from build123d import *

# Parameters (mm, degrees)
ESQUISSE2_W        = 86
ESQUISSE2_H        = 25
ESQUISSE2_R        = 4.05
ESQUISSE2_R_2      = 1
ESQUISSE2_R_3      = 1.5
ESQUISSE2_W_2      = 5
ESQUISSE2_H_2      = 5
BOSS_EXTRU_1_DEPTH = 2
CONG_1_R           = 5


with BuildPart() as part:
    # Esquisse2 → Boss.-Extru.1 (new body)
    with BuildSketch(Plane(origin=(0, 0, 0), x_dir=(-1, 0, 0), z_dir=(0, 0, -1))):
        with Locations((-43, 0)):
            Rectangle(ESQUISSE2_W, ESQUISSE2_H)
        with Locations((-11, 0)):
            Circle(ESQUISSE2_R, mode=Mode.SUBTRACT)
        with Locations((-4, 0)):
            Circle(ESQUISSE2_R_2, mode=Mode.SUBTRACT)
        with Locations((-4.937822174, -3.5)):
            Circle(ESQUISSE2_R_2, mode=Mode.SUBTRACT)
        with Locations((-7.5, -6.062177826)):
            Circle(ESQUISSE2_R_2, mode=Mode.SUBTRACT)
        with Locations((-11, -7)):
            Circle(ESQUISSE2_R_2, mode=Mode.SUBTRACT)
        with Locations((-14.5, -6.062177826)):
            Circle(ESQUISSE2_R_2, mode=Mode.SUBTRACT)
        with Locations((-17.062177826, -3.5)):
            Circle(ESQUISSE2_R_2, mode=Mode.SUBTRACT)
        with Locations((-18, 0)):
            Circle(ESQUISSE2_R_2, mode=Mode.SUBTRACT)
        with Locations((-17.062177826, 3.5)):
            Circle(ESQUISSE2_R_2, mode=Mode.SUBTRACT)
        with Locations((-14.5, 6.062177826)):
            Circle(ESQUISSE2_R_2, mode=Mode.SUBTRACT)
        with Locations((-11, 7)):
            Circle(ESQUISSE2_R_2, mode=Mode.SUBTRACT)
        with Locations((-7.5, 6.062177826)):
            Circle(ESQUISSE2_R_2, mode=Mode.SUBTRACT)
        with Locations((-4.937822174, 3.5)):
            Circle(ESQUISSE2_R_2, mode=Mode.SUBTRACT)
        with Locations((-78.5, 0)):
            Circle(ESQUISSE2_R_3, mode=Mode.SUBTRACT)
        with Locations((-33.7, 0)):
            Circle(ESQUISSE2_R_3, mode=Mode.SUBTRACT)
        with BuildLine():
            Line((-43.7, -2.1), (-58.7, -2.1))
            ThreePointArc((-58.7, -2.1), (-60.8, 0), (-58.7, 2.1))
            Line((-58.7, 2.1), (-43.7, 2.1))
            ThreePointArc((-43.7, 2.1), (-41.6, 0), (-43.7, -2.1))
        make_face(mode=Mode.SUBTRACT)
        with Locations((-78.5, -7.5)):
            Rectangle(ESQUISSE2_W_2, ESQUISSE2_H_2, mode=Mode.SUBTRACT)
        with Locations((-78.5, 7.5)):
            Rectangle(ESQUISSE2_W_2, ESQUISSE2_H_2, mode=Mode.SUBTRACT)
        with Locations((-33.7, -7.5)):
            Rectangle(ESQUISSE2_W_2, ESQUISSE2_H_2, mode=Mode.SUBTRACT)
        with Locations((-33.7, 7.5)):
            Rectangle(ESQUISSE2_W_2, ESQUISSE2_H_2, mode=Mode.SUBTRACT)
    extrude(amount=-BOSS_EXTRU_1_DEPTH)

    # Congé1
    cong_1_edges = [part.edges().sort_by_distance(p)[0] for p in [
        (86, 12.5, 1),
        (0, 12.5, 1),
        (0, -12.5, 1),
        (86, -12.5, 1),
    ]]
    fillet(cong_1_edges, radius=CONG_1_R)


solid = part.part
Read the model definition and answer for the solid it produces. Units are mm, in the model's axes. A direction names the side the tool comes from. Coordinates: 2 decimals unless noted, no trailing zeros. Order: outer loops, then holes, each group sorted by start corner. A loop starts at its lowest first (then second) coordinate and runs counter-clockwise, first axis right, second up. Notation, with made-up numbers: (52.25, 39.5) -> (89.25, 39.5) arc R26 cw to (89.25, 53.5) -> close; hole circle Ø8 at (0.5, 87.25). An arc over 180 degrees is marked (long way). Answer as a JSON object with one key per item and string values.
1) Each of these flat-tipped pins is pushed along its axis until it touches: pin 1 (1.8 mm diameter, centred on x = 4, y = 0, fed in from +Z); pin 2 (4 mm diameter, centred on x = 76.5, y = -8.5, fed in from -Z). Where does it stop, or does it pass through?
Model answer:
{"pin 1": "passes through", "pin 2": "stops at z = 0"}
2) A cutting plane is placed at D-D, the plane z = 1.5. State how many separate pieces and enclosed holes the cut face has, plus the area to 3 significant figures.
Model answer:
{"separate pieces": "1", "enclosed holes": "20", "area": "1,850 mm²"}
3) A tool of negligible diameter and unlimited length cuts with its end or side. For faces 1 (the face through (36.2, 7, 1)), 2 (the face through (44, -12.5, 1)), from which of +Z, -Z, +X, -X, +Y, -Y can it reach the whole face along a straight path? Write none if from no direction.
Model answer:
{"face 1": "+Z, -Z", "face 2": "+Z, -Z, +X, -X, -Y"}
4) A cutting plane is placed at C-C, the plane x = 78.5. Determine the outline of the cut face in (y, z).
Model answer:
{"outline": "(-12.5, 0) -> (-10, 0) -> (-10, 2) -> (-12.5, 2) -> close; (-5, 0) -> (-1.5, 0) -> (-1.5, 2) -> (-5, 2) -> close; (1.5, 0) -> (5, 0) -> (5, 2) -> (1.5, 2) -> close; (10, 0) -> (12.5, 0) -> (12.5, 2) -> (10, 2) -> close"}
5) Consider line 1 along Y through (x, z) = (11, 1.1); line 2 along Y through (x, z) = (36, 0.95); line 3 along X through (y, z) = (-9, 1.85). Determine where each line is inside the solid, lowest interval first. Write a range as from..to.
Model answer:
{"line 1": "y = -12.5..-8, -6..-4.05, 4.05..6, 8..12.5", "line 2": "y = -12.5..-10, -5..5, 10..12.5", "line 3": "x = 0.23..31.2, 36.2..76, 81..85.77"}
6) A cutting plane is placed at B-B, the plane x = 53. Determine the outline of the cut face in (y, z).
Model answer:
{"outline": "(-12.5, 0) -> (-2.1, 0) -> (-2.1, 2) -> (-12.5, 2) -> close; (2.1, 0) -> (12.5, 0) -> (12.5, 2) -> (2.1, 2) -> close"}
7) A cutting plane is placed at A-A, the plane y = 0. Determine the outline of the cut face in (x, z).
Model answer:
{"outline": "(0, 0) -> (3, 0) -> (3, 2) -> (0, 2) -> close; (5, 0) -> (6.95, 0) -> (6.95, 2) -> (5, 2) -> close; (15.05, 0) -> (17, 0) -> (17, 2) -> (15.05, 2) -> close; (19, 0) -> (32.2, 0) -> (32.2, 2) -> (19, 2) -> close; (35.2, 0) -> (41.6, 0) -> (41.6, 2) -> (35.2, 2) -> close; (60.8, 0) -> (77, 0) -> (77, 2) -> (60.8, 2) -> close; (80, 0) -> (86, 0) -> (86, 2) -> (80, 2) -> close"}
8) The mould has two halves that part along X. Classify faces 3 (the face through (1.5, 11.07, 1.01)), 4 (the face through (84.57, 11, 1.01)), 5 (the face through (34, 10, 1)), 6 (the face through (44, -3, 0)): released by +X, released by -X, zero draft, split by the parting line, or undercut.
Model answer:
{"face 3": "released by -X", "face 4": "released by +X", "face 5": "undercut", "face 6": "zero draft"}
